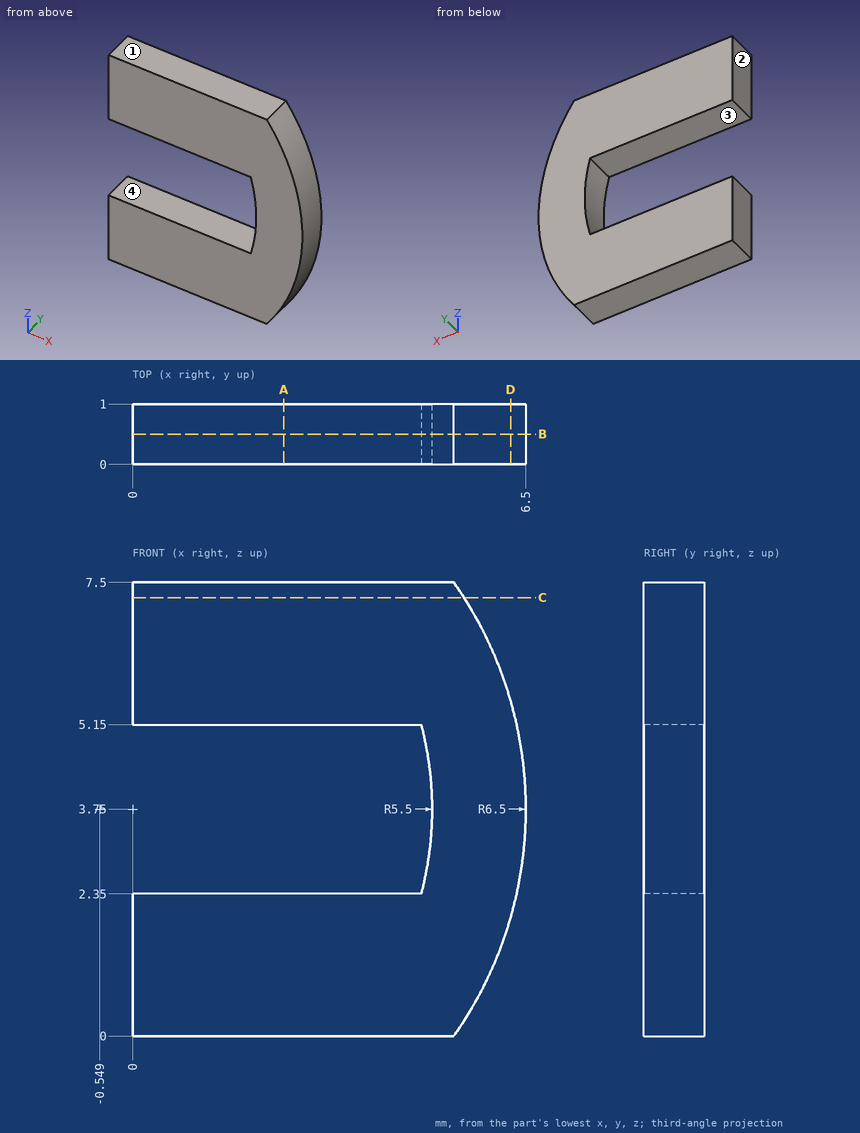
Could you check a few things on this drawing? It's one solid part, dimensions in mm from its lowest x, y, z. Coordinates: 2 decimals unless noted, no trailing zeros. Order: outer loops, then holes, each group sorted by start corner. A loop starts at its lowest first (then second) coordinate and runs counter-clockwise, first axis right, second up.
1. If we section it at A-A (x = 2.5): Please give me the cut outline in (y, z).
2. If we section it at B-B (y = 0.5): Please give me the cut outline in (x, z).
3. If we section it at C-C (z = 7.25): Please give me the cut outline in (x, y).
4. I need wall thicknesses on line 1 (Z direction, x = 2.5, y = 0.4); line 2 (X direction, y = 0.75, z = 3.75); line 3 (X direction, y = 0.25, z = 2). Which ranges of each line are inside material? Lowest first, please.
5. Thinking about a two-plate mould opening in Z: for the marked faces 1, 2, 3 and 4, which applies, +Z half, -Z half, draft (parallel to the pull), parting line (faces both ways), or undercut?
6. I'm going to push a flat-ended pin straight in: pin 1 (1 mm diameter, centred on x = 5, z = 4, fed in from -Y). Where does the tip first touch, or does it pass through?
7. If we section it at D-D (x = 6.25): Please give me the cut outline in (y, z) (1 decimal).
Entries:
1. outline: (0, 0) - (1, 0) - (1, 2.35) - (0, 2.35) - close; (0, 5.15) - (1, 5.15) - (1, 7.5) - (0, 7.5) - close
2. outline: (0, 0) - (5.31, 0) arc R6.5 ccw to (5.31, 7.5) - (0, 7.5) - (0, 5.15) - (4.77, 5.15) arc R5.5 cw to (4.77, 2.35) - (0, 2.35) - close
3. outline: (0, 0) - (5.48, 0) - (5.48, 1) - (0, 1) - close
4. line 1: z = 0 to 2.35, 5.15 to 7.5
4. line 2: x = 4.95 to 6.5
4. line 3: x = 0 to 6.26
5. face 1: +Z half
5. face 2: draft
5. face 3: undercut
5. face 4: undercut
6. pin 1: stops at y = 0
7. outline: (0, 2) - (1, 2) - (1, 5.5) - (0, 5.5) - close
